```python
from build123d import *

# Parameters (mm, degrees)
SKETCH_1_W          = 10
SKETCH_1_H          = 10
SKETCH_1_W_2        = 8
SKETCH_1_H_2        = 8
EXTRUDE_1_DEPTH     = 180
SKETCH_2_R          = 2.1
CUT_EXTRUDE_1_DEPTH = 181.346887969
SKETCH_3_R          = 2.1
CUT_EXTRUDE_2_DEPTH = 181.346887969
SKETCH_4_R          = 1.6
CUT_EXTRUDE_3_DEPTH = 181.346887969
SKETCH_5_R          = 1.6
CUT_EXTRUDE_4_DEPTH = 181.346887969


with BuildPart() as part:
    # ｽｹｯﾁ1 → 押し出し-薄板1 (new body)
    with BuildSketch(Plane(origin=(0, 0, 0), x_dir=(0, 0, -1), z_dir=(1, 0, 0))):
        Rectangle(SKETCH_1_W, SKETCH_1_H)
        Rectangle(SKETCH_1_W_2, SKETCH_1_H_2, mode=Mode.SUBTRACT)
    extrude(amount=EXTRUDE_1_DEPTH)

    # ｽｹｯﾁ2 → ｶｯﾄ - 押し出し1 (cut, through all)
    with BuildSketch(Plane.XY.offset(5)):
        with Locations((7.5, 0)):
            Circle(SKETCH_2_R)
        with Locations(Location((172.5, 0, 0), (0, 0, 90))):
            Circle(SKETCH_2_R)
    extrude(amount=-CUT_EXTRUDE_1_DEPTH, mode=Mode.SUBTRACT)

    # ｽｹｯﾁ3 → ｶｯﾄ - 押し出し2 (cut, through all)
    with BuildSketch(Plane(origin=(0, 5, 0), x_dir=(1, 0, 0), z_dir=(0, 1, 0))):
        with Locations(Location((25, 0, 0), (0, 0, 270))):
            Circle(SKETCH_3_R)
        with Locations(Location((155, 0, 0), (0, 0, 270))):
            Circle(SKETCH_3_R)
    extrude(amount=-CUT_EXTRUDE_2_DEPTH, mode=Mode.SUBTRACT)

    # ｽｹｯﾁ4 → ｶｯﾄ - 押し出し3 (cut, through all)
    with BuildSketch(Plane.XY.offset(5)):
        with Locations((71.7, 0)):
            Circle(SKETCH_4_R)
        with Locations(Location((108.3, 0, 0), (0, 0, 90))):
            Circle(SKETCH_4_R)
    extrude(amount=-CUT_EXTRUDE_3_DEPTH, mode=Mode.SUBTRACT)

    # ｽｹｯﾁ5 → ｶｯﾄ - 押し出し4 (cut, through all)
    with BuildSketch(Plane(origin=(0, 5, 0), x_dir=(1, 0, 0), z_dir=(0, 1, 0))):
        with Locations(Location((57.5, 0, 0), (0, 0, 270))):
            Circle(SKETCH_5_R)
        with Locations(Location((122.5, 0, 0), (0, 0, 270))):
            Circle(SKETCH_5_R)
    extrude(amount=-CUT_EXTRUDE_4_DEPTH, mode=Mode.SUBTRACT)


solid = part.part
```
CAD build for the part. Positions are in the model's coordinates, mm. A direction names the side the tool comes from. Give positions to 0.01 mm unless a question says otherwise; leave off trailing zeros. Order: outer loops, then holes, each group sorted by start corner. A loop starts at its lowest first (then second) coordinate and runs counter-clockwise, first axis right, second up.
(1) Saw through at A-A, the plane x = 68. Give the cut face in (y, z).
(2) Tool access for faces 4 (the flat face through (89, -4, 0)), 5 (the cylindrical face through (157.082, -4.493, -0.273)): list every direction of +Z, -Z, +X, -X, +Y, -Y with a clear straight run to the whole face (end or side of a thin tool).
(3) Saw through at C-C, the plane y = 0. State how many separate pieces and enclosed holes the cut face has, then the cut area to 3 significant figures.
(4) Drill centre lines: L1, parallel to X at y = -4.8, z = 0; L2, parallel to Z at x = 101, y = 1.75; L3, parallel to Z at x = 122.5, y = 4.6. Where is each one in solid material? Low to high.
(5) Flat gauge pin, fed straight in: pin 1 (2.5 mm diameter, centred on x = 57.5, z = 0, fed in from +Y). Where does the tip first touch, or does it go through?
(6) Saw through at B-B, the plane x = 7.5. Give the cut face in (y, z), then the cut area to 3 significant figures.
(7) Mould opens along Z. For faces 1 (the cylindrical face through (70.1, 0.07, 4.51)), 2 (the cylindrical face through (26.77, 4.51, 1.13)), 3 (the flat face through (89, 0, -5)) say: released by +Z, released by -Z, zero draft, split by the parting line, or undercut.
Results found:
1. outline: (-5, -5) - (5, -5) - (5, 5) - (-5, 5) - close; hole (-4, -4) - (4, -4) - (4, 4) - (-4, 4) - close
2. face 4: +X, -X
2. face 5: +Y, -Y
3. separate pieces: 10
3. enclosed holes: 0
3. area: 330 mm2
4. L1: x = 0 to 22.9, 27.1 to 55.9, 59.1 to 120.9, 124.1 to 152.9, 157.1 to 180
4. L2: z = -5 to -4, 4 to 5
4. L3: z = -5 to -1.6, 1.6 to 5
5. pin 1: passes through
6. outline: (-5, -5) - (-2.1, -5) - (-2.1, -4) - (-4, -4) - (-4, 4) - (-2.1, 4) - (-2.1, 5) - (-5, 5) - close; (2.1, -5) - (5, -5) - (5, 5) - (2.1, 5) - (2.1, 4) - (4, 4) - (4, -4) - (2.1, -4) - close
6. area: 27.6 mm2
7. face 1: zero draft
7. face 2: undercut
7. face 3: released by -Z
